from build123d import *

# Parameters (mm, degrees)
F0_R     = 6
F1_DEPTH = 3
F2_DEPTH = 3


with BuildPart() as f1:
    # F0 (on Top) → F1 (new body)
    with BuildSketch(Plane.XY):
        Polygon((-9, 39), (-9, -9), (24, -9), (24, 39), (7.5, 47.554813), align=None)
        Circle(F0_R, mode=Mode.SUBTRACT)
        with Locations((0, 15)):
            Circle(F0_R, mode=Mode.SUBTRACT)
        with Locations((15, 0)):
            Circle(F0_R, mode=Mode.SUBTRACT)
        with Locations((15, 15)):
            Circle(F0_R, mode=Mode.SUBTRACT)
        with Locations((0, 30)):
            Circle(F0_R, mode=Mode.SUBTRACT)
        with Locations((15, 30)):
            Circle(F0_R, mode=Mode.SUBTRACT)
    extrude(amount=F1_DEPTH)

    # F0 (on Top) → F2 (join)
    with BuildSketch(Plane.XY):
        Polygon((-9, 39), (-9, -9), (24, -9), (24, 39), (7.5, 47.554813), align=None)
        Circle(F0_R, mode=Mode.SUBTRACT)
        with Locations((0, 15)):
            Circle(F0_R, mode=Mode.SUBTRACT)
        with Locations((15, 0)):
            Circle(F0_R, mode=Mode.SUBTRACT)
        with Locations((15, 15)):
            Circle(F0_R, mode=Mode.SUBTRACT)
        with Locations((0, 30)):
            Circle(F0_R, mode=Mode.SUBTRACT)
        with Locations((15, 30)):
            Circle(F0_R, mode=Mode.SUBTRACT)
        with Locations((0, 30)):
            Circle(F0_R)
        with Locations((0, 15)):
            Circle(F0_R)
        Circle(F0_R)
        with Locations((15, 0)):
            Circle(F0_R)
        with Locations((15, 15)):
            Circle(F0_R)
        with Locations((15, 30)):
            Circle(F0_R)
    extrude(amount=-F2_DEPTH)


solid = f1.part
Work out the finished part from the listing and answer in its coordinate system (mm). A direction names the side the tool comes from. Round coordinates to 2 decimals unless told otherwise and drop trailing zeros. Loops run counter-clockwise (first coordinate to the right, second up) from the corner with the lowest first, then second, coordinate; pieces in that order, holes last. Notation, with made-up numbers: (-37.75, 53) - (6.25, 53) arc R36 cw to (6.25, 92) - close; hole circle Ø10 at (-24, -38). An arc over 180 degrees is marked (long way). One line per item, written item: value.
Q1. Find section D-D on z = -1.95. Give the vertices of the cut face in (x, y), and give its area (3 significant figures).
Check values:
outline: (-9, -9) - (24, -9) - (24, 39) - (7.5, 47.55) - (-9, 39) - close
area: 1,730 mm2
Q2. The mould has two halves that part along X. Classify faces 3 (the flat face through (15.9, 43.2, 0)), 4 (the flat face through (-0.63, 43.34, 0.04)), 5 (the flat face through (0, 15, 0)), 6 (the flat face through (7, 20, -3)): +X half, -X half, draft (parallel to the pull), parting line (faces both ways), or undercut.
Check values:
face 3: +X half
face 4: -X half
face 5: undercut
face 6: draft
Q3. Find section B-B on y = 0. Give the vertices of the cut face in (x, z).
Check values:
outline: (-9, -3) - (24, -3) - (24, 3) - (21, 3) - (21, 0) - (9, 0) - (9, 3) - (6, 3) - (6, 0) - (-6, 0) - (-6, 3) - (-9, 3) - close
Q4. Find section A-A on z = 0.6. Give the vertices of the cut face in (x, y).
Check values:
outline: (-9, -9) - (24, -9) - (24, 39) - (7.5, 47.55) - (-9, 39) - close; hole circle Ø12 at (0, 0); hole circle Ø12 at (0, 15); hole circle Ø12 at (0, 30); hole circle Ø12 at (15, 0); hole circle Ø12 at (15, 15); hole circle Ø12 at (15, 30)
Q5. For faces 1 (the flat face through (15, 30, 0)), 2 (the flat face through (24, 15, 0)), determine the directions among +Z, -Z, +X, -X, +Y, -Y from which every point of the face is accessible in a straight line to the end or side of a thin tool.
Check values:
face 1: +Z
face 2: +Z, -Z, +X, +Y, -Y
Q6. Each of these flat-tipped pins is pushed along its axis until it touches: pin 1 Ø6 at (x, y) = (14, 1.5) entering from +Z; pin 2 Ø1.5 at (x, z) = (5.5, 1.5) entering from +Y; pin 3 Ø2 at (x, z) = (14, 2) entering from +Y. Where does it stop, or does it pass through?
Check values:
pin 1: z = 0
pin 2: y = 46.91
pin 3: y = 44.7
Q7. Straight lines are drawn through the part: probe 1 along Y at (x, z) = (0, 2.2); probe 2 along Y at (x, z) = (20.5, 1.6); probe 3 along X at (y, z) = (17, 0.9). For each, find the intervals that lie inside material, in ascending order.
Check values:
probe 1: -9 to -6, 6 to 9, 21 to 24, 36 to 43.67
probe 2: -9 to -2.4, 2.4 to 12.6, 17.4 to 27.6, 32.4 to 40.81
probe 3: -9 to -5.66, 5.66 to 9.34, 20.66 to 24
Q8. Find section C-C on x = 0. Give the vertices of the cut face in (y, z), and give its area (3 significant figures).
Check values:
outline: (-9, -3) - (43.67, -3) - (43.67, 3) - (36, 3) - (36, 0) - (24, 0) - (24, 3) - (21, 3) - (21, 0) - (9, 0) - (9, 3) - (6, 3) - (6, 0) - (-6, 0) - (-6, 3) - (-9, 3) - close
area: 208 mm2
